from build123d import *

# Parameters (mm, degrees)
SKETCH1_W           = 100
SKETCH1_H           = 100
BOSS_EXTRUDE1_DEPTH = 60
SKETCH2_W           = 93
SKETCH2_H           = 93
CUT_EXTRUDE1_DEPTH  = 55
SKETCH3_R           = 20
CUT_EXTRUDE2_DEPTH  = 66
FILLET1_R           = 20
FILLET2_R           = 10


with BuildPart() as part:
    # Sketch1 → Boss-Extrude1 (new body)
    with BuildSketch(Plane(origin=(0, 0, 0), x_dir=(1, 0, 0), z_dir=(0, 1, 0))):
        Rectangle(SKETCH1_W, SKETCH1_H)
    extrude(amount=BOSS_EXTRUDE1_DEPTH)

    # Sketch2 → Cut-Extrude1 (cut)
    with BuildSketch(Plane(origin=(0, 60, 0), x_dir=(1, 0, 0), z_dir=(0, 1, 0))):
        Rectangle(SKETCH2_W, SKETCH2_H)
    extrude(amount=-CUT_EXTRUDE1_DEPTH, mode=Mode.SUBTRACT)

    # Sketch3 → Cut-Extrude2 (cut)
    with BuildSketch(Plane(origin=(0, 5, 0), x_dir=(1, 0, 0), z_dir=(0, 1, 0))):
        with Locations(Location((0, 0, 0), (0, 0, 270))):
            Circle(SKETCH3_R)
    extrude(amount=-CUT_EXTRUDE2_DEPTH, mode=Mode.SUBTRACT)

    # Fillet1
    fillet1_edges = [part.edges().sort_by_distance(p)[0] for p in [
        (46.5, 32.5, -46.5),
        (46.5, 32.5, 46.5),
        (-46.5, 32.5, 46.5),
        (-46.5, 32.5, -46.5),
    ]]
    fillet(fillet1_edges, radius=FILLET1_R)

    # Fillet2
    fillet2_edges = [part.edges().sort_by_distance(p)[0] for p in [
        (50, 30, 50),
        (-50, 30, 50),
        (-50, 30, -50),
        (50, 30, -50),
    ]]
    fillet(fillet2_edges, radius=FILLET2_R)


solid = part.part
Could you check a few things on this model? Use its own coordinates, in mm. A direction names the side the tool comes from. Coordinates: 2 decimals unless noted, no trailing zeros. Loops run counter-clockwise (first coordinate to the right, second up) from the corner with the lowest first, then second, coordinate; pieces in that order, holes last.
1. Imagine slicing it at C-C (x = 0). Please give me the cut outline in (y, z).
2. Imagine slicing it at A-A (z = 0). Please give me the cut outline in (x, y).
3. For P1, Ø2, axis at x = -26.5, z = 1.5, coming from the +Y side, with a flat end and sliding along its axis, tell me the tip position at first contact or that it passes through.
4. I need wall thicknesses on L1, parallel to X at y = 26.5, z = -26.5; L2, parallel to X at y = 3, z = 0. Which ranges of each line are inside material? Lowest first, please.
5. For faces 1 (the face through (-40.486, 32.115, -40.797)), 2 (the face through (-1, 30, -50)), which set-ups out of +Z, -Z, +X, -X, +Y, -Y let a thin tool reach every point of the face, with its end or its side?
6. Imagine slicing it at B-B (y = 42). Please give me the cut outline in (x, z), and give its area (3 significant figures).
7. Imagine slicing it at D-D (x = 23). Please give me the cut outline in (y, z).
8. We'd pull the mould along Z, two halves only. Please class faces 3 (the face through (46.99, 30.42, -47.15)), 4 (the face through (-47.15, 30.42, 46.99)), 5 (the face through (46.5, 33, 0)): released by +Z, released by -Z, zero draft, split by the parting line, or undercut.
Computed values:
1. outline: (0, -50) - (60, -50) - (60, -46.5) - (5, -46.5) - (5, -20) - (0, -20) - close; (0, 20) - (5, 20) - (5, 46.5) - (60, 46.5) - (60, 50) - (0, 50) - close
2. outline: (-50, 0) - (-20, 0) - (-20, 5) - (-46.5, 5) - (-46.5, 60) - (-50, 60) - close; (20, 0) - (50, 0) - (50, 60) - (46.5, 60) - (46.5, 5) - (20, 5) - close
3. P1: stops at y = 5
4. L1: x = -50 to -46.5, 46.5 to 50
4. L2: x = -50 to -20, 20 to 50
5. face 1: +Y
5. face 2: -Z, +X, -X, +Y, -Y
6. outline: (-50, -40) arc R10 ccw to (-40, -50) - (40, -50) arc R10 ccw to (50, -40) - (50, 40) arc R10 ccw to (40, 50) - (-40, 50) arc R10 ccw to (-50, 40) - close; hole (-46.5, -26.5) arc R20 ccw to (-26.5, -46.5) - (26.5, -46.5) arc R20 ccw to (46.5, -26.5) - (46.5, 26.5) arc R20 ccw to (26.5, 46.5) - (-26.5, 46.5) arc R20 ccw to (-46.5, 26.5) - close
6. area: 1,610 mm2
7. outline: (0, -50) - (60, -50) - (60, -46.5) - (5, -46.5) - (5, 46.5) - (60, 46.5) - (60, 50) - (0, 50) - close
8. face 3: released by -Z
8. face 4: released by +Z
8. face 5: undercut
